```python
from build123d import *

# Parameters (mm, degrees)
SKETCH_1_W          = 160
SKETCH_1_H          = 80
EXTRUDE_1_DEPTH     = 2
SKETCH_2_R          = 1.3
CUT_EXTRUDE_1_DEPTH = 90.465076985
SKETCH_7_R          = 1.5
CUT_EXTRUDE_3_DEPTH = 90.465076985
FILLET_1_R          = 3


with BuildPart() as part:
    # 草图1 → 凸台-拉伸1 (new body)
    with BuildSketch(Plane.XY):
        Rectangle(SKETCH_1_W, SKETCH_1_H)
    extrude(amount=EXTRUDE_1_DEPTH)

    # 草图2 → 切除-拉伸1 (cut, through all)
    with BuildSketch(Plane.XY.offset(2)):
        with Locations((-33.75, 33)):
            Circle(SKETCH_2_R)
        with Locations((33.75, 33)):
            Circle(SKETCH_2_R)
        with Locations((-22, -23)):
            Circle(SKETCH_2_R)
        with Locations((22, -23)):
            Circle(SKETCH_2_R)
    extrude(amount=-CUT_EXTRUDE_1_DEPTH, mode=Mode.SUBTRACT)

    # 草图7 → 切除-拉伸3 (cut, through all)
    with BuildSketch(Plane(origin=(0, 0, 0), x_dir=(-1, 0, 0), z_dir=(0, 0, -1))):
        with Locations((-70, -30)):
            Circle(SKETCH_7_R)
        with Locations((-70, 30)):
            Circle(SKETCH_7_R)
        with Locations((70, 30)):
            Circle(SKETCH_7_R)
        with Locations((70, -30)):
            Circle(SKETCH_7_R)
    extrude(amount=-CUT_EXTRUDE_3_DEPTH, mode=Mode.SUBTRACT)

    # 圆角1
    fillet_1_edges = [part.edges().sort_by_distance(p)[0] for p in [
        (-80, -40, 1),
        (-80, 40, 1),
        (80, 40, 1),
        (80, -40, 1),
    ]]
    fillet(fillet_1_edges, radius=FILLET_1_R)


solid = part.part
```
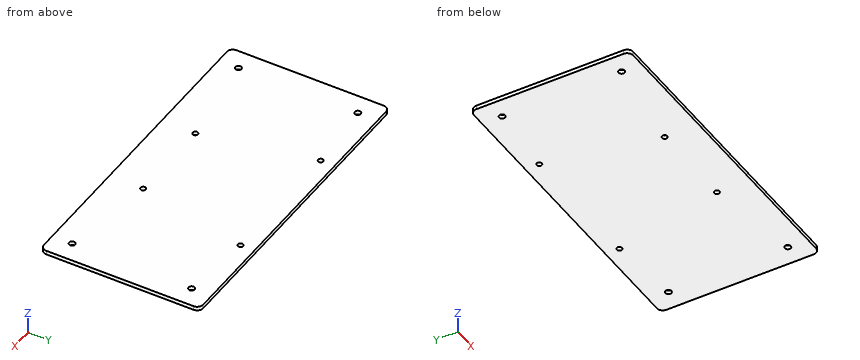
For this review, take the finished solid that the model builds, in its own axes (mm). Give positions to 0.01 mm unless a question says otherwise; leave off trailing zeros. Write each loop counter-clockwise with the first axis right and the second up, starting at its lowest first coordinate (ties: lowest second). Pieces come first, ordered by that corner, then holes.
Item 1: Wall thickness on probe 1 along Y at (x, z) = (-70, 0.8); probe 2 along Y at (x, z) = (33.75, 1.2); probe 3 along Y at (x, z) = (22, 0.5): over which ranges is each line inside the solid? List them lowest first.
Item 2: Take a section at B-B (x = 70). Give the boundary of the cut face in (y, z).
Item 3: Insertion check: P1, Ø2, axis at x = 22, y = -23, coming from the +Z side. The pin has a flat end and moves straight along its axis. Give the tip position at first contact, or say it passes through.
Item 4: Take a section at A-A (y = -30). Give the boundary of the cut face in (x, z), and give its area (3 significant figures).
Established:
1. probe 1: y = -40 to -31.5, -28.5 to 28.5, 31.5 to 40
1. probe 2: y = -40 to 31.7, 34.3 to 40
1. probe 3: y = -40 to -24.3, -21.7 to 40
2. outline: (-40, 0) - (-31.5, 0) - (-31.5, 2) - (-40, 2) - close; (-28.5, 0) - (28.5, 0) - (28.5, 2) - (-28.5, 2) - close; (31.5, 0) - (40, 0) - (40, 2) - (31.5, 2) - close
3. P1: passes through
4. outline: (-80, 0) - (-71.5, 0) - (-71.5, 2) - (-80, 2) - close; (-68.5, 0) - (68.5, 0) - (68.5, 2) - (-68.5, 2) - close; (71.5, 0) - (80, 0) - (80, 2) - (71.5, 2) - close
4. area: 308 mm2
